Job drawing, mm, ordinate dimensions from the low corner. One solid piece. A direction names the side the tool comes from. Give positions to 0.01 mm unless a question says otherwise; leave off trailing zeros. Write each loop counter-clockwise with the first axis right and the second up, starting at its lowest first coordinate (ties: lowest second). Pieces come first, ordered by that corner, then holes. Notation, with made-up numbers: (0.25, 36.25) -> (29.25, 36.25) arc R30 ccw to (29.25, 70.25) -> close; hole circle Ø6 at (-29, 1.5). An arc over 180 degrees is marked (long way). One line per question, with ' | ' between items. Start each with the question number.
(1) Pull direction Z, two halves, no side cores. Call the marked faces 3 and 4: released by +Z, released by -Z, zero draft, split by the parting line, or undercut.
(2) Tool access for the marked faces 1 and 2: list every direction of +Z, -Z, +X, -X, +Y, -Y with a clear straight run to the whole face (end or side of a thin tool).
(3) Band-saw the part on C-C, the plane y = 167. Give the cut face in (x, z).
(4) Band-saw the part on A-A, the plane x = 35.3. Give the cut face in (y, z).
(5) Band-saw the part on B-B, the plane z = 35.3. Give the cut face in (x, y), and give its area (3 significant figures).
(6) Pin check, flat tips, straight feed: P1, Ø1.5, axis at x = 32.5, y = 80, coming from the -Z side; P2, Ø2, axis at y = 63.5, z = 17, coming from the -X side; P3, Ø12, axis at y = 94.5, z = 14, coming from the +X side. Stop position of each tip, or through.
(7) Drill centre lines: probe 1 along X at (y, z) = (164.5, 35.3); probe 2 along X at (y, z) = (47.5, 35.3). Where is each one in solid material? Low to high. Write a range as from..to.
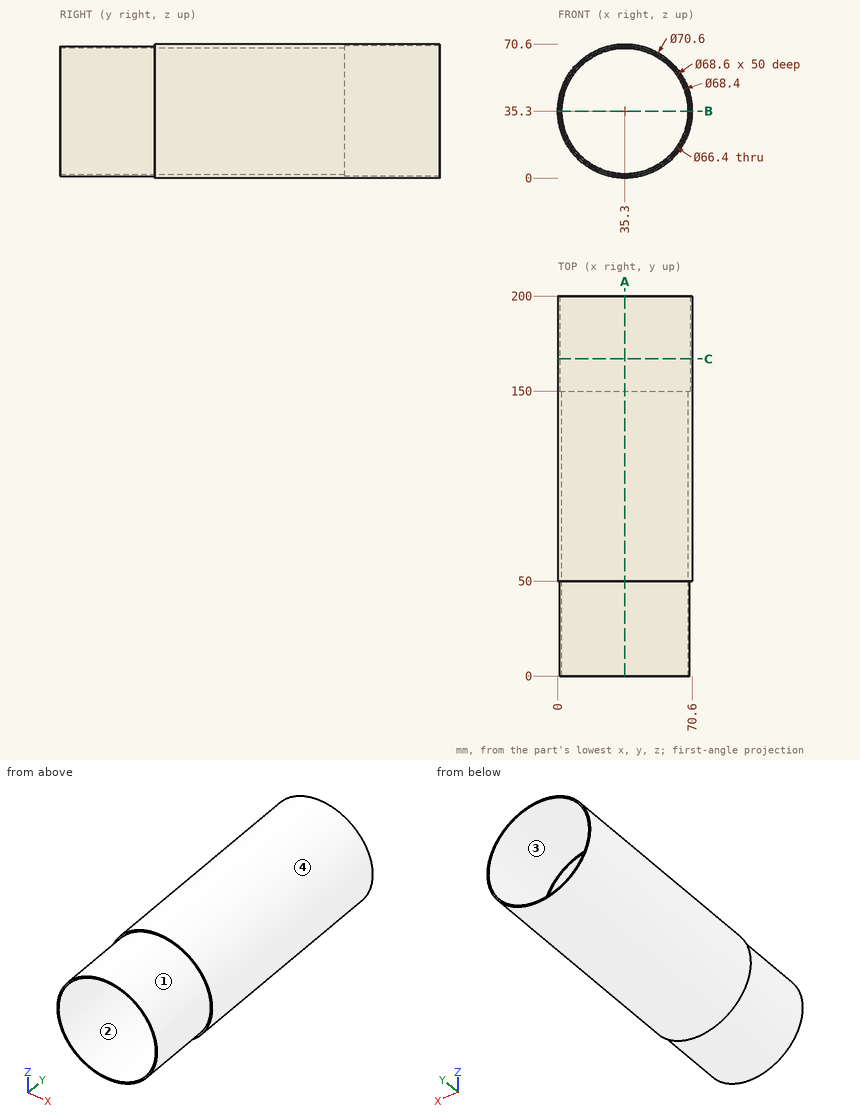
Results:
1) face 3: undercut | face 4: split by the parting line
2) face 1: -Y | face 2: +Y, -Y
3) outline: circle Ø70.6 at (35.3, 35.3); hole circle Ø68.6 at (35.3, 35.3)
4) outline: (0, 1.1) -> (50, 1.1) -> (50, 0) -> (200, 0) -> (200, 1) -> (150, 1) -> (150, 2.1) -> (0, 2.1) -> close; (0, 68.5) -> (150, 68.5) -> (150, 69.6) -> (200, 69.6) -> (200, 70.6) -> (50, 70.6) -> (50, 69.5) -> (0, 69.5) -> close
5) outline: (0, 50) -> (1.1, 50) -> (1.1, 0) -> (2.1, 0) -> (2.1, 150) -> (1, 150) -> (1, 200) -> (0, 200) -> close; (68.5, 0) -> (69.5, 0) -> (69.5, 50) -> (70.6, 50) -> (70.6, 200) -> (69.6, 200) -> (69.6, 150) -> (68.5, 150) -> close | area: 620 mm²
6) P1: stops at z = 0.06 | P2: stops at x = 4.53 | P3: stops at x = 67.11
7) probe 1: x = 0..1, 69.6..70.6 | probe 2: x = 1.1..2.1, 68.5..69.5
